```python
from build123d import *

# Parameters (mm, degrees)
FILLET1_R   = 0.254
HEX_2_DEPTH = 1.6256


with BuildPart() as part:
    # BodySke → Base-Revolve (revolve)
    with BuildSketch(Plane.XY):
        Polygon((0, 0), (0, 2.5146), (0.3556, 2.8702), (3.5052, 2.8702), (3.5052, 1.7526), (41.13276, 1.7526), (41.6052, 1.28016), (41.6052, 0), align=None)
    revolve(axis=Axis((-31.75, 0, 0), (1, 0, 0)))

    # Fillet1
    fillet1_edges = [part.edges().sort_by_distance(p)[0] for p in [
        (3.5052, -1.7526, 0),
    ]]
    fillet(fillet1_edges, radius=FILLET1_R)

    # Sketch2 → Hex-PreBroach (revolve, cut)
    with BuildSketch(Plane.XY):
        Polygon((0, 1.3843), (1.6256, 1.3843), (2.424825978, 0), (0, 0), align=None)
    revolve(axis=Axis((0, 0, 0), (1, 0, 0)), mode=Mode.SUBTRACT)

    # Sketch3 → Hex 2 (cut)
    with BuildSketch(Plane(origin=(0, 0, 0), x_dir=(0, 0.5, 0.866025404), z_dir=(-1, 0, 0))):
        Polygon((0.799225978, 1.3843), (-0.799225978, 1.3843), (-1.598451955, 0), (-0.799225978, -1.3843), (0.799225978, -1.3843), (1.598451955, 0), align=None)
    extrude(amount=-HEX_2_DEPTH, mode=Mode.SUBTRACT)


solid = part.part
```
For this review, take the finished solid that the model builds, in its own axes (mm). A direction names the side the tool comes from. Give positions to 0.01 mm unless a question says otherwise; leave off trailing zeros.
1) For faces 1 (the face through (3.505, 1, 2)), 2 (the face through (0, 0, -2)), 3 (the face through (0.801, 1.193, 0.702)), list the 3-axis set-ups (+Z, -Z, +X, -X, +Y, -Y) from which the entire face can be reached by the end or side of a thin tool; tool diameter is ignored.
2) Insertion check: pin 1 (3 mm diameter, centred on y = 2, z = 2.5, fed in from +X); pin 2 (0.5 mm diameter, centred on x = 0.5, y = -0.5, fed in from -Z); pin 3 (2 mm diameter, centred on x = 5.5, z = 0.5, fed in from -Y); pin 4 (1 mm diameter, centred on y = -2, z = -0.5, fed in from -X). Each pin has a flat end and moves straight along its axis. Give the tip position at first contact, or say it passes through.
3) The part is to be moulded in two halves that separate along Y. For faces 4 (the face through (41.605, 0, 0)), 5 (the face through (1, 0, -1.384)), 6 (the face through (22.71, 1.67, 0.53)), say which applies: released by +Y, released by -Y, zero draft, split by the parting line, or undercut.
4) Wall thickness on line 1 (Z direction, x = 24, y = 0.1); line 2 (X direction, y = 1.55, z = -1.3): over which ranges is each line inside the solid? List them lowest first.
Derived:
1. face 1: +X
1. face 2: +Z, -Z, -X, +Y, -Y
1. face 3: -X
2. pin 1: stops at x = 41.18
2. pin 2: stops at z = -2.86
2. pin 3: stops at y = -1.75
2. pin 4: stops at x = 0
3. face 4: zero draft
3. face 5: undercut
3. face 6: split by the parting line
4. line 1: z = -1.75 to 1.75
4. line 2: x = 0 to 3.51
